Could you check a few things on this model? Use its own coordinates, in mm. A direction names the side the tool comes from. Give positions to 0.01 mm unless a question says otherwise; leave off trailing zeros. Write each loop counter-clockwise with the first axis right and the second up, starting at its lowest first coordinate (ties: lowest second). Pieces come first, ordered by that corner, then holes. Notation, with made-up numbers: M 22,-30.5 L 55,-30.5 A22 ccw 55,-19.5 Z; hole C -22.5,-27 d3. An arc over 180 degrees is marked long. One line per item, written item: value.
```python
from build123d import *

# Parameters (mm, degrees)
ESQUISSE1_W                  = 68.2
ESQUISSE1_H                  = 38.8
BOSS_EXTRU_1_DEPTH           = 1
ESQUISSE3_W                  = 6
ESQUISSE3_H                  = 6
BOSS_EXTRU_2_DEPTH           = 2
ESQUISSE2_W                  = 6
ESQUISSE2_H                  = 6
BOSS_EXTRU_3_DEPTH           = 2
ENL_V_MAT_EXTRU_1_DEPTH      = 79.489999363
ENL_V_MAT_EXTRU_1_DEPTH_BACK = 79.489999363
ESQUISSE5_R                  = 1.75
ESQUISSE6_W                  = 10
ESQUISSE6_H                  = 6
ESQUISSE6_R                  = 1.75
ESQUISSE6_R_2                = 1.8692189
BOSS_EXTRU_4_DEPTH           = 3
ESQUISSE7_W                  = 56.2
ESQUISSE7_H                  = 38.8
BOSS_EXTRU_5_DEPTH           = 4
ESQUISSE8_W                  = 48.2
ESQUISSE8_H                  = 5
BOSS_EXTRU_6_DEPTH           = 20
ESQUISSE9_R                  = 2.25
ENL_V_MAT_EXTRU_2_DEPTH      = 20


with BuildPart() as part:
    # Esquisse1 → Boss.-Extru.1 (new body)
    with BuildSketch(Plane.XY):
        with Locations((34.1, 19.4)):
            Rectangle(ESQUISSE1_W, ESQUISSE1_H)
    extrude(amount=BOSS_EXTRU_1_DEPTH)

    # Esquisse3 → Boss.-Extru.2 (add)
    with BuildSketch(Plane.XY.offset(1)):
        with Locations((65.2, 35.8)):
            Rectangle(ESQUISSE3_W, ESQUISSE3_H)
        with Locations((65.2, 3)):
            Rectangle(ESQUISSE3_W, ESQUISSE3_H)
        with Locations((3, 3)):
            Rectangle(ESQUISSE3_W, ESQUISSE3_H)
    extrude(amount=BOSS_EXTRU_2_DEPTH)

    # Esquisse2 → Boss.-Extru.3 (add)
    with BuildSketch(Plane.XY.offset(1)):
        with Locations((3, 35.8)):
            Rectangle(ESQUISSE2_W, ESQUISSE2_H)
    extrude(amount=BOSS_EXTRU_3_DEPTH)

    # Esquisse5 → Enlèv. mat.-Extru.1 (cut, two sides: drawn at the far end of the back side and taken through both)
    with BuildSketch(Plane.XY.offset(1).offset(-ENL_V_MAT_EXTRU_1_DEPTH_BACK)):
        with Locations((3, 35.8)):
            Circle(ESQUISSE5_R)
        with Locations((3, 3)):
            Circle(ESQUISSE5_R)
        with Locations((65.2, 3)):
            Circle(ESQUISSE5_R)
        with Locations((65.2, 35.8)):
            Circle(ESQUISSE5_R)
    extrude(amount=ENL_V_MAT_EXTRU_1_DEPTH + ENL_V_MAT_EXTRU_1_DEPTH_BACK, mode=Mode.SUBTRACT)

    # Esquisse6 → Boss.-Extru.4 (add)
    # profile 1 of 4: a face of its own
    with BuildSketch(Plane(origin=(0, 0, 0), x_dir=(-1, 0, 0), z_dir=(0, 0, -1))):
        with Locations((-63.2, 3)):
            Rectangle(ESQUISSE6_W, ESQUISSE6_H)
        with Locations(Location((-65.2, 3, 0), (0, 0, 180))):
            Circle(ESQUISSE6_R, mode=Mode.SUBTRACT)
    # profile 2 of 4: a face of its own
    with BuildSketch(Plane(origin=(0, 0, 0), x_dir=(-1, 0, 0), z_dir=(0, 0, -1))):
        with Locations((-63.2, 35.8)):
            Rectangle(ESQUISSE6_W, ESQUISSE6_H)
        with Locations((-65.2, 35.8)):
            Circle(ESQUISSE6_R_2, mode=Mode.SUBTRACT)
    # profile 3 of 4: a face of its own
    with BuildSketch(Plane(origin=(0, 0, 0), x_dir=(-1, 0, 0), z_dir=(0, 0, -1))):
        with Locations((-5, 3)):
            Rectangle(ESQUISSE6_W, ESQUISSE6_H)
        with Locations(Location((-3, 3, 0), (0, 0, 180))):
            Circle(ESQUISSE6_R, mode=Mode.SUBTRACT)
    # profile 4 of 4: a face of its own
    with BuildSketch(Plane(origin=(0, 0, 0), x_dir=(-1, 0, 0), z_dir=(0, 0, -1))):
        with Locations((-5, 35.8)):
            Rectangle(ESQUISSE6_W, ESQUISSE6_H)
        with Locations(Location((-3, 35.8, 0), (0, 0, 180))):
            Circle(ESQUISSE6_R, mode=Mode.SUBTRACT)
    extrude(amount=-BOSS_EXTRU_4_DEPTH)

    # Esquisse7 → Boss.-Extru.5 (add)
    with BuildSketch(Plane(origin=(0, 0, 0), x_dir=(-1, 0, 0), z_dir=(0, 0, -1))):
        with Locations((-34.1, 19.4)):
            Rectangle(ESQUISSE7_W, ESQUISSE7_H)
    extrude(amount=BOSS_EXTRU_5_DEPTH)

    # Esquisse8 → Boss.-Extru.6 (add)
    with BuildSketch(Plane.XZ):
        with Locations((34.1, -1.5)):
            Rectangle(ESQUISSE8_W, ESQUISSE8_H)
    extrude(amount=BOSS_EXTRU_6_DEPTH)

    # Esquisse9 → Enlèv. mat.-Extru.2 (cut)
    with BuildSketch(Plane.XY.offset(1)):
        with BuildLine():
            Line((10, 0), (10, -20))
            Line((10, -20), (30, -20))
            ThreePointArc((30, -20), (16.391056868, -13.608943132), (10, 0))
        make_face()
        with Locations((24, -10)):
            Circle(ESQUISSE9_R)
        with Locations((44.2, -10)):
            Circle(ESQUISSE9_R)
        with BuildLine():
            Line((58.2, -20), (58.2, 0))
            ThreePointArc((58.2, 0), (51.808943132, -13.608943132), (38.2, -20))
            Line((38.2, -20), (58.2, -20))
        make_face()
    extrude(amount=-ENL_V_MAT_EXTRU_2_DEPTH, mode=Mode.SUBTRACT)


solid = part.part
```
1) If we section it at A-A, the plane z = -1.5: Write out the boundary of the cut face in (x, y).
Outcome:
outline: M 6,0 L 10,0 A22.15 ccw 30,-20 L 38.2,-20 A22.15 ccw 58.2,0 L 62.2,0 L 62.2,38.8 L 6,38.8 Z; hole C 24,-10 d4.5; hole C 44.2,-10 d4.5
2) We'd pull the mould along X, two halves only. Please class faces 1 (the face through (63.45, 35.88, 1.48)), 2 (the face through (0, 19.1, 0.8)), 3 (the face through (34, 16, 1)), 4 (the face through (63, 36, 3)): pulls with the +X half, pulls with the -X half, needs draft (parallel to the pull), parting line crosses it, or undercut.
Outcome:
face 1: undercut
face 2: pulls with the -X half
face 3: undercut
face 4: needs draft
3) I'm going to push flat-ended pins straight in: pin 1 (3 mm diameter, centred on y = -3.5, z = -0.5, fed in from -X); pin 2 (1.6 mm diameter, centred on x = 3, z = 1.5, fed in from -Y); pin 3 (4 mm diameter, centred on x = 50.5, z = 1, fed in from -Y). Where does each tip first touch, or does it pass through?
Outcome:
pin 1: stops at x = 10.28
pin 2: stops at y = 0
pin 3: stops at y = -16.33
4) If we section it at B-B, the plane y = 35.8: Write out the boundary of the cut face in (x, z).
Outcome:
outline: M 0,0 L 1.25,0 L 1.25,3 L 0,3 Z; M 4.75,0 L 6,0 L 6,-4 L 62.2,-4 L 62.2,0 L 63.45,0 L 63.45,3 L 58.2,3 L 58.2,1 L 10,1 L 10,3 L 4.75,3 Z; M 66.95,0 L 68.2,0 L 68.2,3 L 66.95,3 Z
5) If we section it at C-C, the plane x = 65.2: Write out the boundary of the cut face in (y, z).
Outcome:
outline: M 0,0 L 1.25,0 L 1.25,3 L 0,3 Z; M 4.75,0 L 34.05,0 L 34.05,3 L 32.8,3 L 32.8,1 L 6,1 L 6,3 L 4.75,3 Z; M 37.55,0 L 38.8,0 L 38.8,3 L 37.55,3 Z
6) If we section it at D-D, the plane x = 7: Write out the boundary of the cut face in (y, z).
Outcome:
outline: M 0,-4 L 38.8,-4 L 38.8,3 L 32.8,3 L 32.8,1 L 6,1 L 6,3 L 0,3 Z
7) On a 3-axis mill with a long thin cutter (end or side, diameter ignored), from which of +Z, -Z, +X, -X, +Y, -Y can I reach the whole of each face in a straight line? I mean faces 5 (the face through (34, 38.8, -1)), 6 (the face through (58.2, 36, 2)), 7 (the face through (62, 0, 0)), 8 (the face through (63, 32.8, 2)). Say none if no direction works.
Outcome:
face 5: +Z, -Z, +X, -X, +Y
face 6: +Z, +Y, -Y
face 7: +Z, -Z, +X, -Y
face 8: +Z, +X, -X
8) Please list where these lines run through material, in increasing order: L1, parallel to X at y = 3, z = 2.45; L2, parallel to Y at x = 65.2, z = 0.9; L3, parallel to Y at x = 3, z = 1.9. Write a range as from..to.
Outcome:
L1: x = 0..1.25, 4.75..10, 58.2..63.45, 66.95..68.2
L2: y = 0..1.25, 4.75..34.05, 37.55..38.8
L3: y = 0..1.25, 4.75..6, 32.8..34.05, 37.55..38.8
